Model file for the job. Use its own axes, mm. Face numbers are marked on the shaded views. A direction names the side the tool comes from. Round coordinates to 2 decimals unless told otherwise and drop trailing zeros. Loops run counter-clockwise (first coordinate to the right, second up) from the corner with the lowest first, then second, coordinate; pieces in that order, holes last.
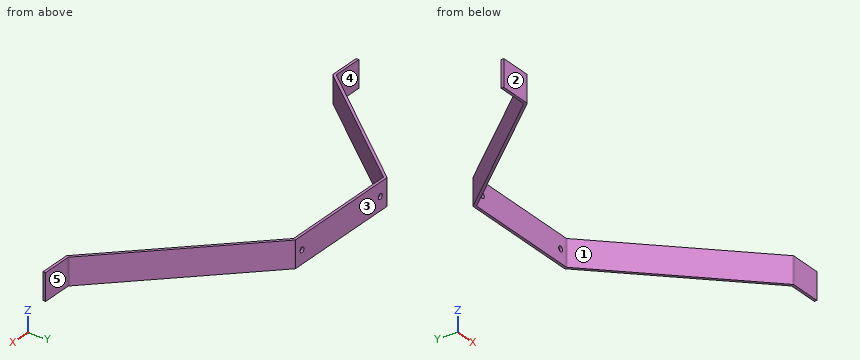
from build123d import *

# Parameters (mm, degrees)
DODANIE_WYCI_GNI_CIE1_DEPTH = 50
ZAOKR_GLENIE1_R             = 2
WYTNIJ_WYCI_GNI_CIE1_REACH  = 841.777
SZKIC2_R                    = 5


with BuildPart() as part:
    # Szkic1 → Dodanie-wyciągnięcie1 (new body)
    with BuildSketch(Plane.XY):
        Polygon((0, 0), (60, 0), (265.92, 245.45), (495.92, 245.45), (740, 0), (800, 0), (800, 5), (742.079269467, 5), (497.999269467, 250.45), (263.588192414, 250.45), (57.668192414, 5), (0, 5), align=None)
    extrude(amount=DODANIE_WYCI_GNI_CIE1_DEPTH)

    # Zaokrąglenie1
    zaokr_glenie1_edges = [part.edges().sort_by_distance(p)[0] for p in [
        (57.668192414, 5, 25),
        (263.588192414, 250.45, 25),
        (497.999269467, 250.45, 25),
        (742.079269467, 5, 25),
        (740, 0, 25),
        (495.92, 245.45, 25),
        (265.92, 245.45, 25),
        (60, 0, 25),
    ]]
    fillet(zaokr_glenie1_edges, radius=ZAOKR_GLENIE1_R)

    # Szkic2 → Wytnij-wyciągnięcie1 (cut, up to next)
    with BuildSketch(Plane(origin=(0, 250.45, 0), x_dir=(1, 0, 0), z_dir=(0, 1, 0)), mode=Mode.PRIVATE) as wytnij_wyci_gni_cie1_sk1:
        with Locations(Location((480.919525398, -24.999999896, 0), (0, 0, 270))):
            Circle(SZKIC2_R)
    wytnij_wyci_gni_cie1_tool1 = extrude(wytnij_wyci_gni_cie1_sk1.sketch, amount=-WYTNIJ_WYCI_GNI_CIE1_REACH, mode=Mode.PRIVATE) & part.part
    # Szkic2 → Wytnij-wyciągnięcie1 (cut, up to next)
    with BuildSketch(Plane(origin=(0, 250.45, 0), x_dir=(1, 0, 0), z_dir=(0, 1, 0)), mode=Mode.PRIVATE) as wytnij_wyci_gni_cie1_sk2:
        with Locations(Location((280.919525398, -24.999999896, 0), (0, 0, 270))):
            Circle(SZKIC2_R)
    wytnij_wyci_gni_cie1_tool2 = extrude(wytnij_wyci_gni_cie1_sk2.sketch, amount=-WYTNIJ_WYCI_GNI_CIE1_REACH, mode=Mode.PRIVATE) & part.part
    add(wytnij_wyci_gni_cie1_tool1.solids().sort_by_distance((480.919525, 250.45, 25))[0], mode=Mode.SUBTRACT)
    add(wytnij_wyci_gni_cie1_tool2.solids().sort_by_distance((280.919525, 250.45, 25))[0], mode=Mode.SUBTRACT)


solid = part.part
Q1. Probe line 1 (X direction, y = 249, z = 25); line 2 (X direction, y = 246, z = 25); line 3 (Y direction, x = 412.5, z = 27). List the from-to ranges inside material, lowest first.
Q2. Flat gauge pins, fed straight in: P1, Ø8, axis at x = 709, z = 44.5, coming from the +Y side; P2, Ø13, axis at x = 280.92, z = 25, coming from the -Y side; P3, Ø4, axis at x = 256, z = 41.5, coming from the -Y side. Where does each tip first touch, or does it go through?
Q3. Slice it at D-D on x = 621.5. Give the cut face in (y, z).
Q4. Tool access for the marked faces 1, 2, 3, 4 and 5: list every direction of +Z, -Z, +X, -X, +Y, -Y with a clear straight run to the whole face (end or side of a thin tool).
Q5. Slice it at B-B on y = 170. Give the cut face in (x, z), plus the area to 3 significant figures.
Q6. Slice it at A-A on z = 43. Give the cut face in (x, y), plus the area to 3 significant figures.
Q7. Slice it at C-C on x = 318. Give the cut face in (y, z).
Reply:
1. line 1: x = 262.37 to 275.92, 285.92 to 475.92, 485.92 to 499.44
1. line 2: x = 259.85 to 275.92, 285.92 to 475.92, 485.92 to 502.42
1. line 3: y = 245.45 to 250.45
2. P1: stops at y = 42.29
2. P2: stops at y = 245.45
2. P3: stops at y = 231.24
3. outline: (119.17, 0) - (126.26, 0) - (126.26, 50) - (119.17, 50) - close
4. face 1: +Z, -Z, -Y
4. face 2: +Z, -Z, +X, -X, -Y
4. face 3: +Z, -Z, +X, -X, +Y
4. face 4: +Z, -Z, -X, +Y
4. face 5: +Z, -Z, +X, +Y
5. outline: (196.09, 0) - (202.62, 0) - (202.62, 50) - (196.09, 50) - close; (570.95, 0) - (578, 0) - (578, 50) - (570.95, 50) - close
5. area: 679 mm2
6. outline: (0, 0) - (59.07, 0) arc R2 ccw to (60.6, 0.71) - (265.32, 244.74) arc R2 cw to (266.85, 245.45) - (495.09, 245.45) arc R2 cw to (496.51, 244.86) - (739.41, 0.59) arc R2 ccw to (740.83, 0) - (800, 0) - (800, 5) - (742.91, 5) arc R2 cw to (741.49, 5.59) - (498.59, 249.86) arc R2 ccw to (497.17, 250.45) - (264.52, 250.45) arc R2 ccw to (262.99, 249.74) - (58.27, 5.71) arc R2 cw to (56.74, 5) - (0, 5) - close
6. area: 5,080 mm2
7. outline: (245.45, 0) - (250.45, 0) - (250.45, 50) - (245.45, 50) - close
